from build123d import *

# Parameters (mm, degrees)
SKETCH1_W           = 23.5
SKETCH1_H           = 28
BOSS_EXTRUDE1_DEPTH = 3.5
CHAMFER1_SIZE       = 1
SKETCH2_R           = 8.5
CUT_EXTRUDE1_DEPTH  = 3.5
SKETCH3_R           = 9.555523526
CUT_EXTRUDE3_DEPTH  = 1
CHAMFER2_SIZE       = 1
SKETCH4_W           = 23.5
SKETCH4_H           = 9.126491789
BOSS_EXTRUDE2_DEPTH = 2
CHAMFER3_SIZE       = 2
CHAMFER4_SIZE       = 1
SKETCH5_W           = 7.502434646
SKETCH5_H           = 2.891999948
CUT_EXTRUDE4_DEPTH  = 1.5
FILLET1_R           = 10
SKETCH6_W           = 23.5
SKETCH6_H           = 2
BOSS_EXTRUDE3_DEPTH = 2
SKETCH7_W           = 25.736202914
SKETCH7_H           = 1.90415655
CUT_EXTRUDE6_DEPTH  = 7
CHAMFER5_SIZE       = 1


# Some blends are built 0.0001 mm under size
with BuildPart() as part:
    # Sketch1 → Boss-Extrude1 (new body)
    with BuildSketch(Plane(origin=(0, 0, 0), x_dir=(1, 0, 0), z_dir=(0, 1, 0))):
        with Locations((-1.454397394, -2.840390879)):
            Rectangle(SKETCH1_W, SKETCH1_H)
    extrude(amount=BOSS_EXTRUDE1_DEPTH)

    # Chamfer1
    chamfer1_edges = [part.edges().sort_by_distance(p)[0] for p in [
        (-1.454397394, 0, -11.159609121),
        (10.295602606, 0, 2.840390879),
        (-13.204397394, 0, 2.840390879),
    ]]
    chamfer(chamfer1_edges, length=CHAMFER1_SIZE)

    # Sketch2 → Cut-Extrude1 (cut)
    with BuildSketch(Plane(origin=(0, 3.5, 0), x_dir=(1, 0, 0), z_dir=(0, 1, 0))):
        with Locations(Location((-1.704397394, -0.840390879, 0), (0, 0, 270))):
            Circle(SKETCH2_R)
    extrude(amount=-CUT_EXTRUDE1_DEPTH, mode=Mode.SUBTRACT)

    # Sketch3 → Cut-Extrude3 (cut)
    with BuildSketch(Plane(origin=(0, 3.5, 0), x_dir=(1, 0, 0), z_dir=(0, 1, 0))):
        with Locations((-1.135292968, 14.156160389)):
            Circle(SKETCH3_R)
    extrude(amount=-CUT_EXTRUDE3_DEPTH, mode=Mode.SUBTRACT)

    # Chamfer2
    chamfer2_edges = [part.edges().sort_by_distance(p)[0] for p in [
        (-8.74141347, 2.5, -8.372134044),
        (6.246016299, 2.5, -8.087857218),
    ]]
    chamfer(chamfer2_edges, length=CHAMFER2_SIZE - 0.0001)  # a hair under: the kernel refuses the full size

    # Sketch4 → Boss-Extrude2 (add)
    with BuildSketch(Plane(origin=(0, 3.5, 0), x_dir=(1, 0, 0), z_dir=(0, 1, 0))):
        with Locations((-1.454397394, -18.777144985)):
            Rectangle(SKETCH4_W, SKETCH4_H)
    extrude(amount=BOSS_EXTRUDE2_DEPTH)

    # Chamfer3
    chamfer3_edges = [part.edges().sort_by_distance(p)[0] for p in [
        (-1.454397394, 3.5, 14.21389909),
    ]]
    chamfer(chamfer3_edges, length=CHAMFER3_SIZE - 0.0001)  # a hair under: the kernel refuses the full size

    # Chamfer4
    chamfer4_edges = [part.edges().sort_by_distance(p)[0] for p in [
        (-1.454397394, 3.5, 16.840390879),
    ]]
    chamfer(chamfer4_edges, length=CHAMFER4_SIZE)

    # Sketch5 → Cut-Extrude4 (cut)
    with BuildSketch(Plane.XZ):
        with Locations((-1.480612468, -6.958763205)):
            Rectangle(SKETCH5_W, SKETCH5_H)
    extrude(amount=-CUT_EXTRUDE4_DEPTH, mode=Mode.SUBTRACT)

    # Fillet1
    # the kernel refuses this fillet: 10 mm, written as the material it takes off along each edge
    with BuildSketch(Plane(origin=(2.270604855, -6.676580089, -6.67288784), x_dir=(0.799474341505259, 0, 0.6007002391165933), z_dir=(0, 1, 0))) as fillet1_piece_1:
        with BuildLine():
            CenterArc((4.241592057, 9.875833363), FILLET1_R, 238.116555861, 22.84506635)
            Line((-1.04033793, 1.384589896), (0, 0))
            ThreePointArc((0, 0), (1.335316018, 0.105541642), (2.670632036, 0))
        make_face()
    extrude(amount=8.176580089, mode=Mode.SUBTRACT)
    with BuildSketch(Plane(origin=(-5.231829791, -6.674182658, -6.89312195), x_dir=(-0.8333660281094135, 0, 0.552721505998401), z_dir=(0, 1, 0))) as fillet1_piece_2:
        with BuildLine():
            CenterArc((4.240068983, -9.875923079), FILLET1_R, 99.035105105, 21.466237943)
            Line((-0.835516616, -1.259750447), (0, 0))
            ThreePointArc((0, 0), (1.334836532, -0.105465383), (2.669673063, 0))
        make_face()
    extrude(amount=8.174182658, mode=Mode.SUBTRACT)

    # Sketch6 → Boss-Extrude3 (add)
    with BuildSketch(Plane.XY.offset(23.340390879)):
        with Locations((-1.454397394, 4.5)):
            Rectangle(SKETCH6_W, SKETCH6_H)
    extrude(amount=BOSS_EXTRUDE3_DEPTH)

    # Sketch7 → Cut-Extrude6 (cut)
    with BuildSketch(Plane(origin=(0, 3.5, 0), x_dir=(1, 0, 0), z_dir=(0, 1, 0))):
        with Locations((-1.767118607, 11.111687396)):
            Rectangle(SKETCH7_W, SKETCH7_H)
    extrude(amount=-CUT_EXTRUDE6_DEPTH, mode=Mode.SUBTRACT)

    # Chamfer5
    chamfer5_edges = [part.edges().sort_by_distance(p)[0] for p in [
        (-1.454397394, 5.5, 25.340390879),
    ]]
    chamfer(chamfer5_edges, length=CHAMFER5_SIZE)


solid = part.part
Design review of the part built by this model. Coordinates are the model's own, in mm. A direction names the side the tool comes from. Coordinates: 2 decimals unless noted, no trailing zeros. Order: outer loops, then holes, each group sorted by start corner. A loop starts at its lowest first (then second) coordinate and runs counter-clockwise, first axis right, second up. Notation, with made-up numbers: M -28.5,8 L -6.5,8 A21 cw -6.5,36 Z; hole C -30,82 d3. An arc over 180 degrees is marked long. Use a Markdown table: item, result.
(1) Add section A-A (z = 5). Give the boundary of the cut face in (x, y).
Worked answers:
| item | result |
|---|---|
| outline | M -13.2,1 L -12.2,0 L -9.12,0 L -9.12,3.5 L -13.2,3.5 Z; M 5.71,0 L 9.3,0 L 10.3,1 L 10.3,3.5 L 5.71,3.5 Z |
(2) For P1, Ø8, axis at x = 6, z = 21.5, coming from the -Y side; P2, Ø1.1, axis at x = -4.5, z = -9, coming from the +Y side; P3, Ø4, axis at x = -10.5, z = 1.5, coming from the +Y side; P4, Ø10, axis at x = 7.5, z = 11, coming from the +Y side, all flat-tipped, find the tip position at first contact; note any pin that passes through.
Worked answers:
| item | result |
|---|---|
| P1 | stops at y = 3.16 |
| P2 | stops at y = 2.5 |
| P3 | stops at y = 3.5 |
| P4 | stops at y = 5.5 |
(3) Add section C-C (z = -3.5). Give the boundary of the cut face in (x, y), then the cut area to 3 significant figures.
Worked answers:
| item | result |
|---|---|
| outline | M -13.2,1 L -12.2,0 L -9.01,0 L -9.01,3.5 L -13.2,3.5 Z; M 5.6,0 L 9.3,0 L 10.3,1 L 10.3,3.5 L 5.6,3.5 Z |
| area | 30.1 mm2 |
(4) Add section D-D (z = 21.5). Give the boundary of the cut face in (x, y).
Worked answers:
| item | result |
|---|---|
| outline | M -13.2,3.5 L 10.3,3.5 L 10.3,5.5 L -13.2,5.5 Z |
(5) For faces 4 (the cylindrical face through (0.849, 1.774, 8.948)), 5 (the flat face through (-1, 2.5, -9)), 6 (the flat face through (-2, 1, 16.84)), 7 (the flat face through (-1, 1.5, -8)), 8 (the flat face through (-2, 1, -10.16)), list the 3-axis set-ups (+Z, -Z, +X, -X, +Y, -Y) from which the entire face can be reached by the end or side of a thin tool; tool diameter is ignored.
Worked answers:
| item | result |
|---|---|
| face 4 | +Y, -Y |
| face 5 | -Z, +Y |
| face 6 | +Z, +X, -X, -Y |
| face 7 | -Y |
| face 8 | -Z, +X, -X, +Y, -Y |
(6) Draft analysis for pull direction X (two halves, no side actions). For faces 1 (the flat face through (9.789, 0.493, 3.529)), 2 (the flat face through (-2, 3.5, 22)), 3 (the conical face through (-7.79, 2.88, -8.19)), state which applies: released by +X, released by -X, zero draft, split by the parting line, or undercut.
Worked answers:
| item | result |
|---|---|
| face 1 | released by +X |
| face 2 | zero draft |
| face 3 | undercut |
(7) Wall thickness on probe 1 along Z at (x, y) = (-6, 1.4); probe 2 along X at (y, z) = (2.55, -2); probe 3 along Z at (x, y) = (1.75, 0.55): over which ranges is each line inside the solid? List them lowest first.
Worked answers:
| item | result |
|---|---|
| probe 1 | z = -10.16 to -7.09, 8.18 to 16.84 |
| probe 2 | x = -13.2 to -9.72, 6.31 to 10.3 |
| probe 3 | z = -10.16 to -8.4, 8.61 to 16.84 |
